```python
from build123d import *

# Parameters (mm, degrees)
F0_W      = 5
F0_H      = 3
F1_DEPTH  = 2
F0_W_2    = 28
F0_H_2    = 7
F2_DEPTH  = 7
F3_D      = 5.5
F5_DEPTH  = 28.001
F6_R      = 3
F7_R      = 5
F8_R      = 0.99999
F9_W      = 4.5
F9_H      = 3.1342408076
F10_DEPTH = 25
F11_D     = 2.3


# Not quite as in the source:
# - a fillet or chamfer is up to 0.001 mm smaller than in the source, because OpenCascade refuses the exact size


with BuildPart() as f1:
    # F0 (on Top) → F1 (new body)
    with BuildSketch(Plane.XY):
        Polygon((-14, -2), (-14, -10), (-4.5, -10), (-4.5, -8), (-2.5, -8), (-2.5, -10), (2.5, -10), (2.5, -8), (4.5, -8), (4.5, -10), (14, -10), (14, -2), align=None)
        with Locations((0, -11.5)):
            Rectangle(F0_W, F0_H)
    extrude(amount=F1_DEPTH)

    # F0 (on Top) → F2 (join)
    with BuildSketch(Plane.XY):
        with Locations((0, 1.5)):
            Rectangle(F0_W_2, F0_H_2)
    extrude(amount=F2_DEPTH)

    # F3 (through all)
    with Locations(Plane(origin=(0, 0, 0), x_dir=(1, 0, 0), z_dir=(0, 0, -1))):
        with Locations((-9.65, 6), (9.65, 6)):
            Hole(F3_D / 2)

    # F4 (on face) → F5 (cut, through all)
    with BuildSketch(Plane.YZ.offset(14)):
        Polygon((5, 7), (-2, 7), (5, 2.9585481157), align=None)
    extrude(amount=-F5_DEPTH, mode=Mode.SUBTRACT)

    # F6
    f6_edges = [f1.edges().sort_by_distance(p)[0] for p in [
        (-14, -10, 1),
        (14, -10, 1),
    ]]
    fillet(f6_edges, radius=F6_R)

    # F7
    f7_edges = [f1.edges().sort_by_distance(p)[0] for p in [
        (14, 5, 1.479274),
        (-14, 5, 1.479274),
    ]]
    fillet(f7_edges, radius=F7_R)

    # F8 (radius 1 in the source; OpenCascade refuses exactly that, so slightly less here)
    f8_edges = [f1.edges().sort_by_distance(p)[0] for p in [
        (0, -2, 7),
        (-4.5, -8, 1),
        (-2.5, -8, 1),
        (2.5, -8, 1),
        (4.5, -8, 1),
        (4.5, -10, 1),
        (-4.5, -10, 1),
        (-2.5, -13, 1),
        (2.5, -13, 1),
    ]]
    fillet(f8_edges, radius=F8_R)

    # F9 (on face) → F10 (cut)
    with BuildSketch(Plane(origin=(0, 2.5310889132, 4.3839745962), x_dir=(1, 0, 0), z_dir=(0, 0.5, 0.8660254038))):
        with BuildLine():
            Line((2.25, 2.8508529611), (-2.25, 2.8508529611))
            Line((-2.25, 2.8508529611), (-2.25, 0.0272258071))
            ThreePointArc((-2.25, 0.0272258071), (0, -2.2227741929), (2.25, 0.0272258071))
            Line((2.25, 0.0272258071), (2.25, 2.8508529611))
        make_face()
        with Locations((0, 4.4179733649)):
            Rectangle(F9_W, F9_H)
    extrude(amount=-F10_DEPTH, mode=Mode.SUBTRACT)

    # F11 (through all)
    with Locations(Plane(origin=(0, 2.5310889132, 4.3839745962), x_dir=(1, 0, 0), z_dir=(0, 0.5, 0.8660254038))):
        with Locations((5.7, 0.0272258071), (-5.7, 0.0272258071)):
            Hole(F11_D / 2)


solid = f1.part
```
Check sheet for the modelled part. Datum: model origin and axes. Units: mm. A direction names the side the tool comes from. Give positions to 0.01 mm unless a question says otherwise; leave off trailing zeros. Order: outer loops, then holes, each group sorted by start corner. A loop starts at its lowest first (then second) coordinate and runs counter-clockwise, first axis right, second up. Notation, with made-up numbers: M -9,58.5 L 1,58.5 A31 cw 1,89.5 Z; hole C 18,20.25 d1. An arc over 180 degrees is marked long. Answer in a Markdown table with one row per item. Add a question column.
Q1. Sectioned sample at C-C, the plane x = 1. Record the boundary of the cut face in (y, z), and give its area (3 significant figures).
Q2. Release check for a two-part mould opening along Y. For faces 4 (the flat face through (8, -10, 1)), 5 (the flat face through (-2.25, 3, 2)), 6 (the cylindrical face through (-5.5, 0.4, 2.9)) record: released by +Y, released by -Y, zero draft, split by the parting line, or undercut.
Q3. Sectioned sample at D-D, the plane x = -6. Record the boundary of the cut face in (y, z).
Q4. Sectioned sample at B-B, the plane x = -9.65. Record the boundary of the cut face in (y, z).
Q5. Sectioned sample at A-A, the plane y = -6. Record the boundary of the cut face in (x, z).
Q6. Access from +Z, -Z, +X, -X, +Y, -Y to the whole of each face (thin tool, end or side, straight path). Record for faces 1 (the flat face through (-6, 5, 1)), 2 (the flat face through (0, -2, 4)), 3 (the cylindrical face through (2.785, -8.301, 1.014)).
Q7. Gauge pin test, flat ends, axial feed: pin 1 Ø5 at (x, y) = (-5.5, -6.5) entering from +Z; pin 2 Ø1.6 at (x, z) = (8.5, 1) entering from -Y; pin 3 Ø3.5 at (x, z) = (3, 3) entering from -Y. Record the tip position at first contact, or that the pin passes through.
Q8. Thickness scan on L1, parallel to X at y = -11.75, z = 0.75; L2, parallel to Y at x = -9.65, z = 1.35; L3, parallel to Z at x = 7.25, y = -8. Record the ranges inside material, lowest first.
Verdict:
| question | item | result |
|---|---|---|
| 1 | outline | M -13,0 L -2.3,0 L 0.81,5.38 L -0.5,6.13 A1 ccw -2,5.27 L -2,2 L -13,2 Z |
| 1 | area | 30.4 mm² |
| 2 | face 4 | released by -Y |
| 2 | face 5 | zero draft |
| 2 | face 6 | undercut |
| 3 | outline | M -10,0 L -1.25,0 L 1.59,4.93 L -0.5,6.13 A1 ccw -2,5.27 L -2,2 L -10,2 Z; M 1.31,0 L 5,0 L 5,2.96 L 3.52,3.82 Z |
| 4 | outline | M -10,0 L -8.75,0 L -8.75,2 L -10,2 Z; M -3.25,0 L 4.96,0 L 4.96,2.98 L -0.5,6.13 A1 ccw -2,5.27 L -2,2 L -3.25,2 Z |
| 5 | outline | M -14,0 L -12.4,0 L -12.4,2 L -14,2 Z; M -6.9,0 L 6.9,0 L 6.9,2 L -6.9,2 Z; M 12.4,0 L 14,0 L 14,2 L 12.4,2 Z |
| 6 | face 1 | +Z, -Z, +X, -X, +Y |
| 6 | face 2 | +Z, +X, -X, -Y |
| 6 | face 3 | +Z, -Z, -Y |
| 7 | pin 1 | z = 2 |
| 7 | pin 2 | y = -10 |
| 7 | pin 3 | y = -13 |
| 8 | L1 | -2.5 to 2.5 |
| 8 | L2 | -10 to -8.75, -3.25 to 4.96 |
| 8 | L3 | 0 to 2 |
